The model under review builds one solid part; all positions refer to its coordinate system, in mm. A direction names the side the tool comes from. Coordinates: 2 decimals unless noted, no trailing zeros. Loops run counter-clockwise (first coordinate to the right, second up) from the corner with the lowest first, then second, coordinate; pieces in that order, holes last. Notation, with made-up numbers: M 44.5,29.25 L 70.5,29.25 A29 cw 70.5,60.25 Z; hole C -39,79 d8. An arc over 180 degrees is marked long. Write item = value, one per line. Start each with the question number.
Q1. We need section A-A on x = 7. Give the boundary of the cut face in (y, z).
Q2. We need section C-C on y = 46. Give the boundary of the cut face in (x, z), and give its area (3 significant figures).
Q3. Clearance check with flat-ended pins moving along their axes: pin 1 Ø1.5 at (x, z) = (15.5, 13.5) entering from +Y; pin 2 Ø1.5 at (x, z) = (30, 25) entering from +Y; pin 3 Ø6 at (y, z) = (16.5, 25) entering from +X. State where each tip first meets the part, or that it passes through.
Q4. For faces 4 (the face through (8, 45.7, 18.4)), 5 (the face through (0.99, 16.81, 32.34)), 6 (the face through (25, 2, 44)), 7 (the face through (26, 46, 4)), 8 (the face through (15.38, 11.29, 0.99)), list the 3-axis set-ups (+Z, -Z, +X, -X, +Y, -Y) from which the entire face can be reached by the end or side of a thin tool; tool diameter is ignored.
Q5. Mouldability with a two-part tool opening along Y and no side actions: class faces 1 (the face through (45, 24, 1)), 2 (the face through (6, 10, 36)), 3 (the face through (26, 7, 16)) as released by +Y, released by -Y, zero draft, split by the parting line, or undercut.
Q6. Wall thickness on probe 1 along X at (y, z) = (16, 4.65); probe 2 along Y at (x, z) = (16, 0.55); probe 3 along Y at (x, z) = (16, 1.35): over which ranges is each line inside the solid? List them lowest first.
Q7. We need section D-D on x = 46. Give the boundary of the cut face in (y, z).
Q8. We need section B-B on z = 4.5. Give the boundary of the cut face in (x, y), and give its area (3 significant figures).
from build123d import *

# Parameters (mm, degrees)
F1_DEPTH  = 6
F3_DEPTH  = 20
F5_DEPTH  = 40
F7_DEPTH  = 60
F9_DEPTH  = 2
F11_DEPTH = 2
F13_DEPTH = 2
F14_R     = 2.25
F15_DEPTH = 8
F16_R     = 2.25
F17_DEPTH = 8
F18_R     = 3.25
F18_R_2   = 2.25
F19_DEPTH = 8.001
F20_R     = 3.75
F21_DEPTH = 2
F22_R     = 3.75
F23_DEPTH = 2
F24_R     = 3.75
F24_R_2   = 4.75
F25_DEPTH = 2
F26_SIZE  = 3


with BuildPart() as f1:
    # F0 (on Top) → F1 (new body)
    with BuildSketch(Plane.XY):
        Polygon((0, 66), (0, 0), (66, 0), (66, 26), (26, 26), (26, 66), align=None)
    extrude(amount=F1_DEPTH)

    # F2 (on face) → F3 (join)
    with BuildSketch(Plane.XY.offset(6)):
        Polygon((6, 66), (0, 66), (0, 0), (66, 0), (66, 6), (6, 6), align=None)
    extrude(amount=F3_DEPTH)

    # F4 (on face) → F5 (join)
    with BuildSketch(Plane.XY.offset(26)):
        Polygon((6, 6), (6, 26), (0, 26), (0, 0), (26, 0), (26, 6), align=None)
    extrude(amount=F5_DEPTH)

    # F6 (on face) → F7 (join)
    with BuildSketch(Plane.XY.offset(6)):
        Polygon((13.29, 6), (16, 6), (18.71, 6), (18.71, 8), (13.29, 8), align=None)
        Polygon((6, 18.71), (6, 16), (6, 13.29), (8, 13.29), (8, 18.71), align=None)
    extrude(amount=F7_DEPTH)

    # F8 (on face) → F9 (join)
    with BuildSketch(Plane.XY.offset(6)):
        Polygon((66, 13.29), (66, 16), (66, 18.71), (26, 18.71), (26, 13.29), align=None)
        Polygon((18.71, 66), (16, 66), (13.29, 66), (13.29, 26), (18.71, 26), align=None)
    extrude(amount=F9_DEPTH)

    # F10 (on face) → F11 (join)
    with BuildSketch(Plane(origin=(0, 6, 0), x_dir=(-1, 0, 0), z_dir=(0, 1, 0))):
        Polygon((-66, 18.71), (-66, 16), (-66, 13.29), (-26, 13.29), (-26, 16), (-26, 18.71), align=None)
    extrude(amount=F11_DEPTH)

    # F12 (on face) → F13 (join)
    with BuildSketch(Plane.YZ.offset(6)):
        Polygon((66, 13.29), (66, 16), (66, 18.71), (26, 18.71), (26, 13.29), align=None)
    extrude(amount=F13_DEPTH)

    # F14 (on face) → F15 (cut, through all)
    with BuildSketch(Plane.XZ):
        with Locations((56, 16)):
            Circle(F14_R)
        with Locations((16, 46)):
            Circle(F14_R)
        with Locations((36, 16)):
            Circle(F14_R)
    extrude(amount=-F15_DEPTH, mode=Mode.SUBTRACT)

    # F16 (on face) → F17 (cut, through all)
    with BuildSketch(Plane(origin=(0, 0, 0), x_dir=(0, -1, 0), z_dir=(-1, 0, 0))):
        with Locations((-16, 56)):
            Circle(F16_R)
        with Locations((-46, 16)):
            Circle(F16_R)
        with Locations((-16, 36)):
            Circle(F16_R)
    extrude(amount=-F17_DEPTH, mode=Mode.SUBTRACT)

    # F18 (on face) → F19 (cut, through all)
    with BuildSketch(Plane(origin=(0, 0, 0), x_dir=(1, 0, 0), z_dir=(0, 0, -1))):
        with Locations((16, -16)):
            Circle(F18_R)
        with Locations((46, -16)):
            Circle(F18_R_2)
        with Locations((16, -56)):
            Circle(F18_R_2)
        with Locations((16, -36)):
            Circle(F18_R_2)
    extrude(amount=-F19_DEPTH, mode=Mode.SUBTRACT)

    # F20 (on face) → F21 (cut)
    with BuildSketch(Plane.XZ):
        with Locations((16, 46)):
            Circle(F20_R)
        with Locations((36, 16)):
            Circle(F20_R)
        with Locations((56, 16)):
            Circle(F20_R)
    extrude(amount=-F21_DEPTH, mode=Mode.SUBTRACT)

    # F22 (on face) → F23 (cut)
    with BuildSketch(Plane(origin=(0, 0, 0), x_dir=(0, -1, 0), z_dir=(-1, 0, 0))):
        with Locations((-16, 56)):
            Circle(F22_R)
        with Locations((-46, 16)):
            Circle(F22_R)
        with Locations((-16, 36)):
            Circle(F22_R)
    extrude(amount=-F23_DEPTH, mode=Mode.SUBTRACT)

    # F24 (on face) → F25 (cut)
    with BuildSketch(Plane(origin=(0, 0, 0), x_dir=(1, 0, 0), z_dir=(0, 0, -1))):
        with Locations((16, -56)):
            Circle(F24_R)
        with Locations((16, -16)):
            Circle(F24_R_2)
        with Locations((46, -16)):
            Circle(F24_R)
        with Locations((16, -36)):
            Circle(F24_R)
    extrude(amount=-F25_DEPTH, mode=Mode.SUBTRACT)

    # F26
    f26_edges = [f1.edges().sort_by_distance(p)[0] for p in [
        (33, 0, 0),
        (0, 33, 0),
        (0, 0, 33),
        (0, 26, 46),
        (0, 46, 26),
        (26, 0, 46),
        (46, 0, 26),
        (0, 13, 66),
        (13, 0, 66),
        (0, 66, 13),
        (13, 66, 0),
        (66, 0, 13),
        (66, 13, 0),
        (46, 26, 0),
        (26, 46, 0),
    ]]
    chamfer(f26_edges, length=F26_SIZE)


solid = f1.part
Returned:
q1.outline = M 0,3 L 3,0 L 63,0 L 66,3 L 66,6 L 18.71,6 L 18.71,66 L 13.29,66 L 13.29,6 L 6,6 L 6,66 L 3,66 L 0,63 Z; M 26,13.29 L 66,13.29 L 66,18.71 L 26,18.71 Z; hole C 16,36 d4.5; hole C 16,56 d4.5; hole C 46,16 d4.5
q2.outline = M 0,3 L 3,0 L 23,0 L 26,3 L 26,6 L 18.71,6 L 18.71,8 L 13.29,8 L 13.29,6 L 6,6 L 6,13.29 L 8,13.29 L 8,13.75 L 2,13.75 L 2,12.25 L 0,12.25 Z; M 0,19.75 L 2,19.75 L 2,18.25 L 8,18.25 L 8,18.71 L 6,18.71 L 6,26 L 3,26 L 0,23 Z
q2.area = 242 mm^2
q3.pin_1 = 8
q3.pin_2 = 6
q3.pin_3 = 8
q4.face_4 = +Z, +X, +Y
q4.face_5 = -X
q4.face_6 = +Z, +X, -Y
q4.face_7 = +Z, -Z, +X, +Y
q4.face_8 = -Z
q5.face_1 = released by +Y
q5.face_2 = undercut
q5.face_3 = zero draft
q6.probe_1 = 0 to 12.75, 19.25 to 43.75, 48.25 to 66
q6.probe_2 = 2.45 to 11.25, 20.75 to 32.25, 39.75 to 52.25, 59.75 to 63.55
q6.probe_3 = 1.65 to 11.25, 20.75 to 32.25, 39.75 to 52.25, 59.75 to 64.35
q7.outline = M 0,3 L 3,0 L 12.25,0 L 12.25,2 L 13.75,2 L 13.75,8 L 13.29,8 L 13.29,6 L 6,6 L 6,13.29 L 8,13.29 L 8,18.71 L 6,18.71 L 6,26 L 3,26 L 0,23 Z; M 18.25,2 L 19.75,2 L 19.75,0 L 23,0 L 26,3 L 26,6 L 18.71,6 L 18.71,8 L 18.25,8 Z
q8.outline = M 0,3 L 3,0 L 63,0 L 66,3 L 66,26 L 26,26 L 26,66 L 3,66 L 0,63 Z; hole C 16,16 d6.5; hole C 16,36 d4.5; hole C 16,56 d4.5; hole C 46,16 d4.5
q8.area = 2,660 mm^2
